Geometry: final body of the model. Coordinates: model frame, mm. Face numbers are marked on the shaded views. A direction names the side the tool comes from. Give positions to 0.01 mm unless a question says otherwise; leave off trailing zeros. Loops run counter-clockwise (first coordinate to the right, second up) from the corner with the lowest first, then second, coordinate; pieces in that order, holes last.
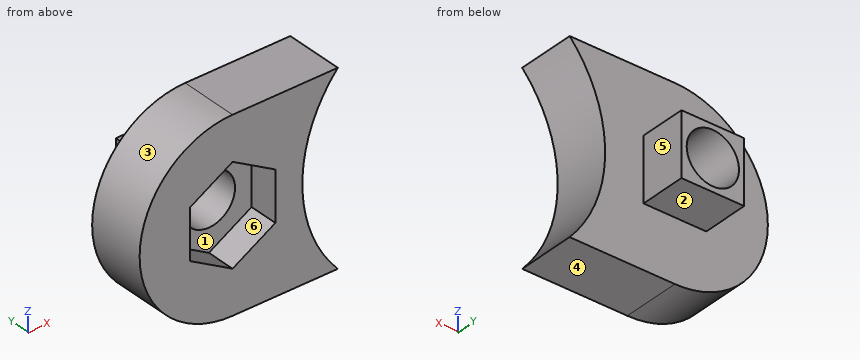
from build123d import *

# Parameters (mm, degrees)
PAD023_DEPTH      = 5
BOX003_W          = 5.4
BOX003_H          = 5.4
BOX003_DEPTH      = 4
CYLINDER064_R     = 2.25
CYLINDER064_DEPTH = 9
POCKET005_DEPTH   = 2.5


with BuildPart() as part:
    # Sketch033 → Pad023 (new body)
    with BuildSketch(Plane.XZ):
        with BuildLine():
            ThreePointArc((-18, 8), (-26, 0), (-18, -8))
            Line((-18, -8), (-8.944272, -8))
            ThreePointArc((-8.944272, 8), (-12, 0), (-8.944272, -8))
            Line((-18, 8), (-8.944272, 8))
        make_face()
    extrude(amount=PAD023_DEPTH)

    # Box003 → Box003 (join)
    with BuildSketch(Plane(origin=(-20.7, 4, -2.7), x_dir=(1, 0, 0), z_dir=(0, -1, 0))):
        with Locations((2.7, 2.7)):
            Rectangle(BOX003_W, BOX003_H)
    extrude(amount=BOX003_DEPTH)

    # Cylinder064 → Cylinder064 (cut)
    with BuildSketch(Plane(origin=(-18, 4, 0), x_dir=(1, 0, 0), z_dir=(0, -1, 0))):
        Circle(CYLINDER064_R)
    extrude(amount=CYLINDER064_DEPTH, mode=Mode.SUBTRACT)

    # Sketch035 (on Face5 of Cylinder064) → Pocket005 (cut)
    with BuildSketch(Plane(origin=(-18, -5, 0), x_dir=(1, 0, 0), z_dir=(0, -1, 0))):
        Polygon((3.680608, 2.125), (0, 4.25), (-3.680608, 2.125), (-3.680608, -2.125), (0, -4.25), (3.680608, -2.125), align=None)
    extrude(amount=-POCKET005_DEPTH, mode=Mode.SUBTRACT)


with BuildPart() as part_1:
    # Body035 placement: moved
    add(part.part.moved(Location((0, -5, 0))))


solid = part_1.part
Item 1: Section query A-A on z = 0. Return loops of the section in (x, y).
Values follow:
outline: (-26, -10) - (-21.68, -10) - (-21.68, -7.5) - (-20.25, -7.5) - (-20.25, -1) - (-20.7, -1) - (-20.7, -5) - (-26, -5) - close; (-15.75, -7.5) - (-14.32, -7.5) - (-14.32, -10) - (-12, -10) - (-12, -5) - (-15.3, -5) - (-15.3, -1) - (-15.75, -1) - close
Item 2: Draft query along Z for the marked faces 4, 5 and 6. Return one class per face: +Z half, -Z half, draft (parallel to the pull), parting line (faces both ways), or undercut.
Values follow:
face 4: -Z half
face 5: draft
face 6: undercut
Item 3: Section query B-B on x = -19. Return loops of the section in (y, z), plus the area to 3 significant figures.
Values follow:
outline: (-10, -7.94) - (-5, -7.94) - (-5, -2.7) - (-1, -2.7) - (-1, -2.02) - (-7.5, -2.02) - (-7.5, -3.67) - (-10, -3.67) - close; (-10, 3.67) - (-7.5, 3.67) - (-7.5, 2.02) - (-1, 2.02) - (-1, 2.7) - (-5, 2.7) - (-5, 7.94) - (-10, 7.94) - close
area: 56.4 mm2
Item 4: Ray query, probe 1 along X at (y, z) = (-4.25, 0); probe 2 along Z at (x, y) = (-18, -4.5); probe 3 along X at (y, z) = (-6, 0). Return the intervals inside material, ascending.
Values follow:
probe 1: x = -20.7 to -20.25, -15.75 to -15.3
probe 2: z = -2.7 to -2.25, 2.25 to 2.7
probe 3: x = -26 to -20.25, -15.75 to -12
Item 5: Section query D-D on y = -4. Return loops of the section in (x, z), plus the area to 3 significant figures.
Values follow:
outline: (-20.7, -2.7) - (-15.3, -2.7) - (-15.3, 2.7) - (-20.7, 2.7) - close; hole circle Ø4.5 at (-18, 0)
area: 13.3 mm2
Item 6: Section query C-C on y = -8. Return loops of the section in (x, z) (3 decimals), plus the area to 3 significant figures.
Values follow:
outline: (-18, -8) - (-8.944, -8) arc R12 cw to (-8.944, 8) - (-18, 8) arc R8 ccw to start; hole (-21.681, -2.125) - (-18, -4.25) - (-14.319, -2.125) - (-14.319, 2.125) - (-18, 4.25) - (-21.681, 2.125) - close
area: 165 mm2
Item 7: Pin query (flat end, axial travel): pin 1 (1.5 mm diameter, centred on x = -16, y = -2.5, fed in from +Z); pin 2 (1.5 mm diameter, centred on y = -8, z = 3, fed in from +X); pin 3 (5 mm diameter, centred on x = -18, z = 0, fed in from -Y). Return the tip coordinate at first contact, or that it passes through.
Values follow:
pin 1: stops at z = 2.7
pin 2: stops at x = -11.4
pin 3: stops at y = -7.5
Item 8: Set-up query: the marked faces 1, 2 and 3. Return all of +Z, -Z, +X, -X, +Y, -Y with unobstructed straight access to the full face (end or side cutting, diameter ignored); none if empty.
Values follow:
face 1: -Y
face 2: -Z, +X, -X, +Y
face 3: -X, +Y, -Y
